```python
from build123d import *

# Parameters (mm, degrees)
BOSS_EXTRUDE1_DEPTH         = 12.7
F_1_4_20_TAPPED_HOLE1_D     = 5.1054
F_3_16_0_1875_DOWEL_HOLE1_D = 4.7625


with BuildPart() as part:
    # Sketch1 → Boss-Extrude1 (new body, symmetric)
    with BuildSketch(Plane(origin=(0, 0, 0), x_dir=(0, 0, -1), z_dir=(1, 0, 0))):
        Polygon((8.89, -95.25), (8.89, 22.225), (-19.685, 22.225), (-19.685, 0), (0, 0), (0, -95.25), align=None)
    extrude(amount=BOSS_EXTRUDE1_DEPTH, both=True)

    # Sketch2 → Cut-Revolve4 (revolve, cut)
    with BuildSketch(Plane(origin=(0, 0, 0), x_dir=(0, 0, -1), z_dir=(1, 0, 0))):
        Polygon((-26.697108117, 5.566910104), (-3.81, 21.592635735), (-3.81, 22.225), (-26.697108117, 22.225), align=None)
    revolve(axis=Axis((0, 21.592635735, 3.81), (0, 1, 0)), mode=Mode.SUBTRACT)

    # 1/4-20 Tapped Hole1 (through all)
    with Locations(Plane(origin=(0, 0, 0), x_dir=(-1, 0, 0), z_dir=(0, -1, 0))):
        with Locations((0, -13.335)):
            Hole(F_1_4_20_TAPPED_HOLE1_D / 2)

    # 3/16 (0.1875) Dowel Hole1 (through all)
    with Locations(Plane(origin=(12.7, 0, 0), x_dir=(0, 0, -1), z_dir=(1, 0, 0))):
        with Locations((4.1275, -88.9), (4.1275, -69.85)):
            Hole(F_3_16_0_1875_DOWEL_HOLE1_D / 2)


solid = part.part
```
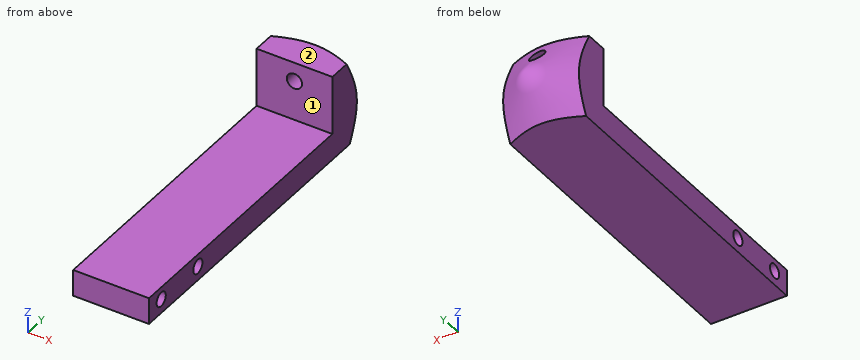
Work out the finished part from the listing and answer in its coordinate system (mm). Face numbers are marked on the shaded views. A direction names the side the tool comes from. Round coordinates to 2 decimals unless told otherwise and drop trailing zeros. Write each loop counter-clockwise with the first axis right and the second up, starting at its lowest first coordinate (ties: lowest second). Pieces come first, ordered by that corner, then holes. Notation, with made-up numbers: (-11, 69) - (6, 69) arc R8 ccw to (6, 75) - close; hole circle Ø7 at (-12, 26.5). An arc over 180 degrees is marked (long way). Return JSON: item names as keys, results as strings. Group by question number.
Q1. For the marked faces 1 and 2, determine the directions among +Z, -Z, +X, -X, +Y, -Y from which every point of the face is accessible in a straight line to the end or side of a thin tool.
Q2. Each of these flat-tipped pins is pushed along its axis until it touches: pin 1 Ø12 at (x, z) = (2, 15.5) entering from -Y; pin 2 Ø1.5 at (x, z) = (-5.5, -4) entering from +Y; pin 3 Ø3 at (y, z) = (-69.85, -4.13) entering from +X; pin 4 Ø6 at (x, z) = (0, 13.335) entering from +Y. Where does it stop, or does it pass through?
Q3. Find the intervals of material crossed by L1, parallel to Y at x = 2.5, z = -5.5; L2, parallel to Y at x = 0.25, z = -3.25; L3, parallel to Z at x = 0.5, y = -69, in increasing order.
Q4. The part is cut by section A-A on y = -69.85. Write down the section's boundary in (x, z).
Q5. The part is cut by section B-B on x = 1. Count the separate pieces of the cut face and the enclosed holes in it, then the cut area to 3 significant figures.
Solved:
{
 "1": {"face 1": "+Z, +X, -X, -Y", "face 2": "+Z, +X, -X, +Y, -Y"},
 "2": {"pin 1": "y = 0", "pin 2": "y = 15.43", "pin 3": "through", "pin 4": "y = 17.02"},
 "3": {"L1": "-95.25 to -90.85, -86.95 to -71.8, -67.9 to 14.84", "L2": "-95.25 to -91.11, -86.69 to -72.06, -67.64 to 16.65", "L3": "-8.89 to -6.35, -1.9 to 0"},
 "4": {"outline": "(-12.7, -8.89) - (12.7, -8.89) - (12.7, -6.51) - (-12.7, -6.51) - close; (-12.7, -1.75) - (12.7, -1.75) - (12.7, 0) - (-12.7, 0) - close"},
 "5": {"separate pieces": "2", "enclosed holes": "2", "area": "1,210 mm²"}
}
